The listing builds one solid part. Answer for the finished solid, in the listing's coordinates (mm). Face numbers are marked on the shaded views. A direction names the side the tool comes from. Coordinates: 2 decimals unless noted, no trailing zeros. Order: outer loops, then holes, each group sorted by start corner. A loop starts at its lowest first (then second) coordinate and runs counter-clockwise, first axis right, second up. Notation, with made-up numbers: (70, 65) -> (94, 65) arc R19 ccw to (94, 77) -> close; hole circle Ø8 at (72, 9). An arc over 180 degrees is marked (long way). One line per question, with ' | ' between items.
Autodesk Fusion 360 part; units mm, degrees
sketch "Sketch1" plane through (0, 0, 0) normal (0, 0, 1) x (1, 0, 0)
  circle A0 centre (0, 0) radius 35
  circle A1 centre (0, 0) radius 38
  line L0 (-38, 0) -> (-38, 38)
  line L1 (-38, 38) -> (0, 38)
  line L2 (0, 1.75) -> (0, 22.5)
  line L3 (38, 38) -> (0, 38)
  line L4 (38, 0) -> (38, 38)
  line L5 (2.0599, 34.9393) -> (2.0599, 2)
  line L6 (2.0599, -2) -> (2.0599, -34.9393)
  line L7 (-34.9428, 2) -> (-1.9401, 2)
  line L8 (2.0599, 2) -> (34.9428, 2)
  line L9 (-1.9401, 34.9462) -> (-1.9401, 2)
  line L10 (-1.9401, -2) -> (-1.9401, -34.9462)
  line L11 (-34.9428, -2) -> (-1.9401, -2)
  line L12 (2.0599, -2) -> (34.9428, -2)
  dimension "d1" = 70
  dimension "d2" = 3
  dimension "d27" = 38
  dimension "d28" = 38
extrude "Extrude1" add sketch "Sketch1" along normal blind 3 contours A0 L5 L6 L7 L8 L9 L10 L11 L12 | A1 | A1 L3 L4 | A1 L0 L1
sketch "Sketch3" plane through (0, 38, 0) normal (0, 1, 0) x (-1, 0, 0)
  line L0 (-38, 0) -> (38, 0)
  line L1 (38, 0) -> (38, 3)
  line L2 (38, 3) -> (-38, 3)
  line L3 (-38, 0) -> (38, 0)
  line L4 (38, 0) -> (38, 60)
  line L5 (38, 60) -> (0, 60)
  circle A0 centre (-20, 45) radius 2
  circle A1 centre (0, 45) radius 2
  circle A2 centre (20, 45) radius 2
  line L6 (-38, 60) -> (0, 60)
  line L7 (-38, 0) -> (-38, 60)
  line L8 (-38, 0) -> (38, 0)
  line L9 (-38, 3) -> (-38, 0)
  dimension "d9" = 60
  dimension "d10" = 38
  dimension "d11" = 4
extrude "Extrude4" add sketch "Sketch3" along normal blind 3 contours L2 L4 L5 L6 L7
extrude "Extrude5" add sketch "Sketch1" along normal blind 30
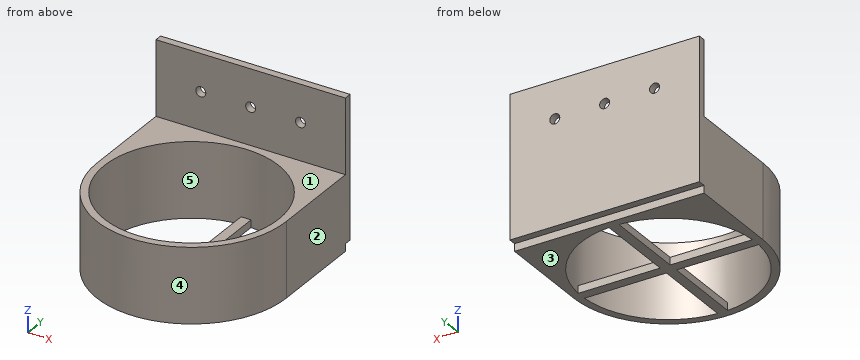
Item 1: Section A-A, the plane x = 8.5 is taken. Give the vertices of the cut face in (y, z).
Computed values:
outline: (-37.04, 0) -> (-33.95, 0) -> (-33.95, 30) -> (-37.04, 30) -> close; (-2, 0) -> (2, 0) -> (2, 3) -> (-2, 3) -> close; (33.95, 0) -> (38, 0) -> (38, 3) -> (41, 3) -> (41, 60) -> (38, 60) -> (38, 30) -> (33.95, 30) -> close
Item 2: For the marked faces 1 and 2, determine the directions among +Z, -Z, +X, -X, +Y, -Y from which every point of the face is accessible in a straight line to the end or side of a thin tool.
Computed values:
face 1: +Z, +X, -X, -Y | face 2: +Z, -Z, +X, +Y, -Y
Item 3: Section D-D, the plane z = 45 is taken. Give the vertices of the cut face in (x, y).
Computed values:
outline: (-38, 38) -> (-22, 38) -> (-22, 41) -> (-38, 41) -> close; (-18, 38) -> (-2, 38) -> (-2, 41) -> (-18, 41) -> close; (2, 38) -> (18, 38) -> (18, 41) -> (2, 41) -> close; (22, 38) -> (38, 38) -> (38, 41) -> (22, 41) -> close
Item 4: Section C-C, the plane x = -0.5 is taken. Give the vertices of the cut face in (y, z), plus the area to 3 significant figures.
Computed values:
outline: (-38, 0) -> (38, 0) -> (38, 3) -> (41, 3) -> (41, 43.06) -> (38, 43.06) -> (38, 30) -> (35, 30) -> (35, 3) -> (-35, 3) -> (-35, 30) -> (-38, 30) -> close; (38, 46.94) -> (41, 46.94) -> (41, 60) -> (38, 60) -> close | area: 549 mm^2
Item 5: Find the intervals of material crossed by L1, parallel to Y at x = 0, z = 24.25; L2, parallel to X at y = 0, z = 6; L3, parallel to Z at x = 0, y = 39.95, in increasing order.
Computed values:
L1: y = -38 to -35, 35 to 41 | L2: x = -38 to -35, 35 to 38 | L3: z = 3 to 43, 47 to 60
Item 6: Determine the mould class of the marked faces 3, 4 and 5 for opening direction X: pulls with the +X half, pulls with the -X half, needs draft (parallel to the pull), parting line crosses it, or undercut.
Computed values:
face 3: needs draft | face 4: parting line crosses it | face 5: undercut
Item 7: Each of these flat-tipped pins is pushed along its axis until it touches: pin 1 Ø3.5 at (x, z) = (-21, 2) entering from -Y; pin 2 Ø8 at (x, z) = (-7.5, 50) entering from -Y; pin 3 Ø21 at (x, y) = (-11.5, -9.5) entering from +Z. Where does it stop, or does it pass through?
Computed values:
pin 1: stops at y = -32.76 | pin 2: stops at y = 38 | pin 3: stops at z = 3
Item 8: Section B-B, the plane z = 20.5 is taken. Give the vertices of the cut face in (x, y).
Computed values:
outline: (-38, 0) arc R38 ccw to (38, 0) -> (38, 41) -> (-38, 41) -> close; hole circle Ø70 at (0, 0)
